```python
from build123d import *

# Parameters (mm, degrees)
SKETCH1_W              = 63.5
SKETCH1_H              = 101.6
BOSS_EXTRUDE1_DEPTH    = 6.35
SKETCH3_R              = 8.73125
CUT_EXTRUDE1_DEPTH     = 3.81
F_8_CLEARANCE_HOLE2_D  = 4.4958
SKETCH4_R              = 7.9375
CUT_EXTRUDE2_DEPTH     = 7.9375
FILLET1_R              = 6.35
F_10_CLEARANCE_HOLE1_D = 5.1054
CUT_EXTRUDE3_DEPTH     = 3.175
FILLET2_R              = 3.175
SKETCH11_R             = 4.445
CUT_EXTRUDE4_DEPTH     = 2.286


with BuildPart() as part:
    # Sketch1 → Boss-Extrude1 (new body)
    with BuildSketch(Plane(origin=(0, 0, 0), x_dir=(1, 0, 0), z_dir=(0, 1, 0))):
        Rectangle(SKETCH1_W, SKETCH1_H)
    extrude(amount=BOSS_EXTRUDE1_DEPTH)

    # Sketch3 → Cut-Extrude1 (cut)
    with BuildSketch(Plane(origin=(0, 6.35, 0), x_dir=(1, 0, 0), z_dir=(0, 1, 0))):
        with Locations((0, 10.16)):
            Circle(SKETCH3_R)
    extrude(amount=-CUT_EXTRUDE1_DEPTH, mode=Mode.SUBTRACT)

    # #8 Clearance Hole2 (through all)
    with Locations(Plane(origin=(0, 0, 0), x_dir=(-1, 0, 0), z_dir=(0, -1, 0))):
        with Locations((-4.7, 24.00000002), (4.7, -23.99999998), (4.7, 24.00000002), (-4.7, -23.99999998)):
            Hole(F_8_CLEARANCE_HOLE2_D / 2)

    # Sketch4 → Cut-Extrude2 (cut)
    with BuildSketch(Plane.XZ):
        with Locations((0, -10.16)):
            Circle(SKETCH4_R)
    extrude(amount=-CUT_EXTRUDE2_DEPTH, mode=Mode.SUBTRACT)

    # Fillet1
    fillet1_edges = [part.edges().sort_by_distance(p)[0] for p in [
        (-31.75, 3.175, -50.8),
        (31.75, 3.175, -50.8),
        (31.75, 3.175, 50.8),
        (-31.75, 3.175, 50.8),
    ]]
    fillet(fillet1_edges, radius=FILLET1_R)

    # #10 Clearance Hole1 (through all)
    with Locations(Plane(origin=(0, 6.35, 0), x_dir=(1, 0, 0), z_dir=(0, 1, 0))):
        with Locations((25.4, 44.45), (-25.4, 44.45), (-25.4, -44.45), (25.4, -44.45), (-25.4, 0), (25.4, 0)):
            Hole(F_10_CLEARANCE_HOLE1_D / 2)

    # Sketch10 → Cut-Extrude3 (cut)
    with BuildSketch(Plane.XZ):
        with BuildLine():
            Line((19.05, -44.45), (-19.05, -44.45))
            ThreePointArc((-19.05, -44.45), (-20.909871939, -39.959871939), (-25.4, -38.1))
            Line((-25.4, -38.1), (-25.4, -6.35))
            ThreePointArc((-25.4, -6.35), (-19.05, 0), (-25.4, 6.35))
            Line((-25.4, 6.35), (-25.4, 38.1))
            ThreePointArc((-25.4, 38.1), (-20.909871939, 39.959871939), (-19.05, 44.45))
            Line((-19.05, 44.45), (19.05, 44.45))
            ThreePointArc((19.05, 44.45), (20.909871939, 39.959871939), (25.4, 38.1))
            Line((25.4, 38.1), (25.4, 6.35))
            ThreePointArc((25.4, 6.35), (19.05, 0), (25.4, -6.35))
            Line((25.4, -6.35), (25.4, -38.1))
            ThreePointArc((25.4, -38.1), (20.909871939, -39.959871939), (19.05, -44.45))
        make_face()
        with BuildLine():
            ThreePointArc((0, -24.769029441), (7.830394623, -27.589155318), (6.100677898, -19.448131428))
            ThreePointArc((6.100677898, -19.448131428), (0, 0.9525), (-6.100677898, -19.448131428))
            ThreePointArc((-6.100677898, -19.448131428), (-7.830394623, -27.589155318), (0, -24.769029441))
        make_face(mode=Mode.SUBTRACT)
        with BuildLine():
            ThreePointArc((0, 23.230970559), (9.4625, 23.99999998), (0, 24.769029401))
            ThreePointArc((0, 24.769029401), (-9.4625, 23.99999998), (0, 23.230970559))
        make_face(mode=Mode.SUBTRACT)
    extrude(amount=-CUT_EXTRUDE3_DEPTH, mode=Mode.SUBTRACT)

    # Fillet2
    fillet2_edges = [part.edges().sort_by_distance(p)[0] for p in [
        (25.4, 1.5875, -38.1),
        (19.05, 1.5875, -44.45),
        (-19.05, 1.5875, -44.45),
        (-25.4, 1.5875, -38.1),
        (-25.4, 1.5875, -6.35),
        (-25.4, 1.5875, 6.35),
        (-25.4, 1.5875, 38.1),
        (-19.05, 1.5875, 44.45),
        (19.05, 1.5875, 44.45),
        (25.4, 1.5875, 38.1),
        (25.4, 1.5875, 6.35),
        (25.4, 1.5875, -6.35),
        (-6.100677898, 1.5875, -19.448131428),
        (6.100677898, 1.5875, -19.448131428),
        (0, 1.5875, -24.769029441),
        (0, 1.5875, 24.769029401),
        (0, 1.5875, 23.230970559),
    ]]
    fillet(fillet2_edges, radius=FILLET2_R)

    # Sketch11 → Cut-Extrude4 (cut)
    with BuildSketch(Plane(origin=(0, 6.35, 0), x_dir=(1, 0, 0), z_dir=(0, 1, 0))):
        with Locations((4.7, -23.99999998)):
            Circle(SKETCH11_R)
        with Locations((-4.7, -23.99999998)):
            Circle(SKETCH11_R)
        with Locations((4.7, 24.00000002)):
            Circle(SKETCH11_R)
        with Locations((-4.7, 24.00000002)):
            Circle(SKETCH11_R)
    extrude(amount=-CUT_EXTRUDE4_DEPTH, mode=Mode.SUBTRACT)


solid = part.part
```
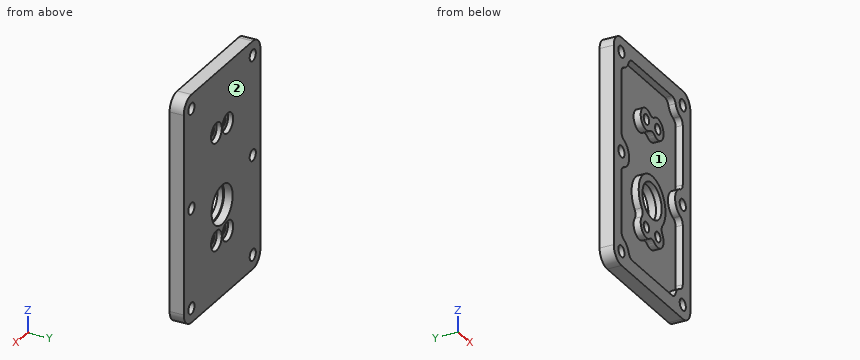
The model under review builds one solid part; all positions refer to its coordinate system, in mm. Face numbers are marked on the shaded views. Round coordinates to 2 decimals unless told otherwise and drop trailing zeros. Loops run counter-clockwise (first coordinate to the right, second up) from the corner with the lowest first, then second, coordinate; pieces in that order, holes last. Notation, with made-up numbers: M 26,19.5 L 41,19.5 A36 ccw 41,53.5 Z; hole C 89.5,56.25 d3. An arc over 180 degrees is marked long. Put each result on its own line as item: value.
Q1. For pin 1 (4 mm diameter, centred on x = 25.4, z = -44.45, fed in from -Y); pin 2 (4.5 mm diameter, centred on x = -3, z = 24.5, fed in from +Y); pin 3 (10 mm diameter, centred on x = 18.5, z = -27.5, fed in from -Y) (3 decimals), all flat-tipped, find the tip position at first contact; note any pin that passes through.
Result set:
pin 1: passes through
pin 2: stops at y = 4.06
pin 3: stops at y = 3.175
Q2. Consider section C-C, the plane x = -17.5. Give the boundary of the cut face in (y, z) (3 decimals), then the cut area to 3 significant figures.
Result set:
outline: M 0,-50.8 L 6.35,-50.8 L 6.35,50.8 L 0,50.8 L 0,44.261 L 3.175,44.261 L 3.175,-44.261 L 0,-44.261 Z
area: 364 mm²
Q3. Mouldability with a two-part tool opening along Z and no side actions: class the marked faces 1 and 2 as released by +Z, released by -Z, zero draft, split by the parting line, or undercut.
Result set:
face 1: undercut
face 2: zero draft
Q4. Consider section A-A, the plane z = 24. Count the separate pieces of the cut face and the enclosed holes in it, then the cut area to 3 significant figures.
Result set:
separate pieces: 3
enclosed holes: 0
area: 225 mm²
Q5. To check wall thickness, follow L1, parallel to X at y = 5, z = 24 (3 decimals); L2, parallel to X at y = 4, z = 24; L3, parallel to Z at x = -25.4, y = 3.75. State the ranges of each line that lie inside material, in increasing order.
Result set:
L1: x = -31.75 to -9.145, -0.255 to 0.255, 9.145 to 31.75
L2: x = -31.75 to -6.95, -2.45 to 2.45, 6.95 to 31.75
L3: z = -50.8 to -47, -41.9 to -2.55, 2.55 to 41.9, 47 to 50.8
